Verification items for the finished model (mm, model axes). A direction names the side the tool comes from. Coordinates: 2 decimals unless noted, no trailing zeros. Loops run counter-clockwise (first coordinate to the right, second up) from the corner with the lowest first, then second, coordinate; pieces in that order, holes last. Notation, with made-up numbers: (-32, -14) - (13, -14) arc R32 ccw to (13, 20) - close; hole circle Ø10 at (11, 62). An arc over 180 degrees is marked (long way). One line per item, written item: value. Start each with the question number.
(1) Thickness scan on probe 1 along Z at (x, y) = (15.9, 3.25); probe 2 along X at (y, z) = (3, 16); probe 3 along Z at (x, y) = (-15.9, 1.15). Record the ranges inside material, lowest first. Write a range as [from, to].
(2) Section check B-B (z = 35). Record the boundary of the cut face in (x, y), plus the area to 3 significant figures.
(3) Draft check along X on faces 5 (the face through (0, 0, 24)), 6 (the face through (-21.9, 3, 24)), 7 (the face through (2.493, 32.127, 8.028)). Enter one of: +X half, -X half, draft (parallel to the pull), parting line (faces both ways), or undercut.
(4) Set-up check for faces 1 (the face through (0, 6, 24)), 2 (the face through (14.1, 25, 8)), 3 (the face through (-14, 2, 37)), 4 (the face through (-14.114, 0.986, 17.369)): record each of +Z, -Z, +X, -X, +Y, -Y from which the full face is reachable in a straight line by a thin tool's end or side.
(5) Section check A-A (y = 20.9). Record the boundary of the cut face in (x, z), plus the area to 3 significant figures.
(6) Section check C-C (x = -15). Record the boundary of the cut face in (y, z).
(7) Section check D-D (z = 24). Record the boundary of the cut face in (x, y), plus the area to 3 significant figures.
(8) Gauge pin test, flat ends, axial feed: P1, Ø6, axis at x = 15.9, z = 35, coming from the -Y side; P2, Ø10.5, axis at x = 15.9, z = 16, coming from the +Y side; P3, Ø8.5, axis at x = -8, y = 24.5, coming from the +Z side; P4, Ø4, axis at x = 16.5, z = 16.5, coming from the +Y side. Record the tip position at first contact, or that the pin passes through.
Autodesk Inventor part; units mm, degrees
ref_plane "YZ Plane" through (0, 0, 0) normal (1, 0, 0) x (0, 1, 0)
ref_plane "XZ Plane" through (0, 0, 0) normal (0, 1, 0) x (-1, 0, 0)
ref_plane "XY Plane" through (0, 0, 0) normal (0, 0, 1) x (1, 0, 0)
sketch "Sketch1" plane through (0, 0, 0) normal (0, 1, 0) x (-1, 0, 0)
  circle A0 centre (15.9, 35) radius 2.25
  circle A1 centre (15.9, 16) radius 2.25
  circle A2 centre (-15.9, 16) radius 2.25
  circle A3 centre (-15.9, 35) radius 2.25
  line L0 (21.9, 10) -> (-21.9, 10)
  line L1 (-21.9, 10) -> (-21.9, 41)
  line L2 (-21.9, 41) -> (21.9, 41)
  line L3 (21.9, 41) -> (21.9, 10)
  point P0 (0, 0)
  point P1 (0, 0)
  dimension "d0" = 43.8
  dimension "d1" = 31
extrude "Extrusion1" add sketch "Sketch1" along normal blind 6
sketch "Sketch2" plane through (0, 6, 0) normal (0, 1, 0) x (1, 0, 0)
  circle A0 centre (-15.9, -16) radius 2.25
  circle A1 centre (-15.9, -16) radius 4
  circle A2 centre (-15.9, -35) radius 2.25
  circle A3 centre (-15.9, -35) radius 4
  circle A4 centre (15.9, -35) radius 2.25
  circle A5 centre (15.9, -35) radius 4
  circle A6 centre (15.9, -16) radius 2.25
  circle A7 centre (15.9, -16) radius 4
  point P0 (0, 0)
  dimension "d4" = 8
  dimension "d5" = 8
  dimension "d6" = 8
  dimension "d7" = 8
extrude "Extrusion2" cut sketch "Sketch2" against normal blind 4
sketch "Sketch4" plane through (21.9, 0, 10) normal (0, 0, -1) x (-1, 0, 0)
  line L0 (43.8, 0) -> (0, 0)
  line L1 (43.8, 0) -> (43.8, 6)
  line L2 (0, 6) -> (43.8, 6)
  line L3 (0, 0) -> (0, 6)
  line L4 (0, 6) -> (43.8, 6)
  line L5 (36, 6) -> (36, 35)
  line L6 (36, 35) -> (21.9, 35)
  line L7 (36, 35) -> (7.8, 35)
  line L8 (7.8, 35) -> (7.8, 6)
  line L9 (36, 6.8) -> (36, 35)
  line L10 (33.4, 32.4) -> (21.9, 32.4)
  line L11 (10.4, 9.4) -> (33.4, 9.4)
  circle A0 centre (33.4, 32.4) radius 1.75
  circle A1 centre (10.4, 32.4) radius 1.75
  circle A2 centre (10.4, 9.4) radius 1.75
  circle A3 centre (33.4, 9.4) radius 1.75
  circle A4 centre (21.9, 20.9) radius 11.5
  point P0 (21.9, 0)
  dimension "d31" = 14.1
  dimension "d34" = 11.5
  dimension "d39" = 3.5
  dimension "d40" = 3.5
  dimension "d41" = 3.5
  dimension "d42" = 3.5
  dimension "d43" = 23
extrude "Extrusion4" add sketch "Sketch4" along normal blind 4
chamfer "Chamfer3" distance 7.8 angle 45 1 edges at (14.1, 6, 8)
chamfer "Chamfer4" distance 7.8 angle 45 1 edges at (-14.1, 6, 8)
properties part number "NEMA14 Mounting Bracket"
Responses:
1. probe 1: z = [6, 12], [20, 31], [39, 41]
1. probe 2: x = [-21.9, -19.9], [-11.9, 11.9], [19.9, 21.9]
1. probe 3: z = [6, 13.75], [18.25, 32.75], [37.25, 41]
2. outline: (-21.9, 0) - (-18.15, 0) - (-18.15, 2) - (-19.9, 2) - (-19.9, 6) - (-21.9, 6) - close; (-13.65, 0) - (13.65, 0) - (13.65, 2) - (11.9, 2) - (11.9, 6) - (-11.9, 6) - (-11.9, 2) - (-13.65, 2) - close; (18.15, 0) - (21.9, 0) - (21.9, 6) - (19.9, 6) - (19.9, 2) - (18.15, 2) - close
2. area: 181 mm²
3. face 5: draft
3. face 6: -X half
3. face 7: undercut
4. face 1: +Z, +X, -X, +Y
4. face 2: +Z, -Z, +X, +Y
4. face 3: +Y
4. face 4: +Y, -Y
5. outline: (-14.1, 6) - (-11.5, 6) - (-11.5, 10) - (-14.1, 10) - close; (11.5, 6) - (14.1, 6) - (14.1, 10) - (11.5, 10) - close
5. area: 20.8 mm²
6. outline: (0, 6) - (12.9, 6) - (12.9, 10) - (6, 10) - (6, 12.1) - (2, 12.1) - (2, 13.94) - (0, 13.94) - close; (0, 18.06) - (2, 18.06) - (2, 19.9) - (6, 19.9) - (6, 31.1) - (2, 31.1) - (2, 32.94) - (0, 32.94) - close; (0, 37.06) - (2, 37.06) - (2, 38.9) - (6, 38.9) - (6, 41) - (0, 41) - close
7. outline: (-21.9, 0) - (21.9, 0) - (21.9, 6) - (-21.9, 6) - close
7. area: 263 mm²
8. P1: stops at y = 0
8. P2: stops at y = 6
8. P3: stops at z = 10
8. P4: stops at y = 2
